```python
from build123d import *

# Parameters (mm, degrees)
BOSS_EXTRUDE1_DEPTH = 1.5


with BuildPart() as part:
    # Sketch1 → Boss-Extrude1 (new body)
    with BuildSketch(Plane(origin=(0, 0, 0), x_dir=(1, 0, 0), z_dir=(0, 1, 0))):
        with BuildLine():
            Line((15, 0), (4.75, 0))
            Line((4.75, 0), (4.75, 2))
            Line((4.75, 2), (-4.75, 2))
            Line((-4.75, 2), (-4.75, 0))
            Line((-4.75, 0), (-15, 0))
            Line((-15, 0), (-25.356589319, -6.472868325))
            ThreePointArc((-25.356589319, -6.472868325), (-27.468846161, -12.236329652), (-33.575081251, -11.609425782))
            Line((-33.575081251, -11.609425782), (-71, -35))
            Line((-71, -35), (-89.017448096, -62.257165069))
            ThreePointArc((-89.017448096, -62.257165069), (-90.820615058, -63.903738488), (-93.18854397, -64.5))
            Line((-93.18854397, -64.5), (-115.5, -64.5))
            Line((-115.5, -64.5), (-116, -65))
            Line((-116, -65), (-116, -155))
            Line((-116, -155), (-89.131068486, -155))
            ThreePointArc((-89.131068486, -155), (-86.477376272, -154.23767833), (-84.632870889, -152.183167051))
            Line((-84.632870889, -152.183167051), (-59, -99.369197466))
            Line((-59, -99.369197466), (-59, -77.369197466))
            ThreePointArc((-59, -77.369197466), (-54, -72.369197466), (-49, -77.369197466))
            Line((-49, -77.369197466), (-49, -104.800858216))
            ThreePointArc((-49, -104.800858216), (-44, -109.800858216), (-39, -104.800858216))
            Line((-39, -104.800858216), (-39, -82.800858216))
            ThreePointArc((-39, -82.800858216), (0, -43.800858216), (39, -82.800858216))
            Line((39, -82.800858216), (39, -104.800858216))
            ThreePointArc((39, -104.800858216), (44, -109.800858216), (49, -104.800858216))
            Line((49, -104.800858216), (49, -77.369197466))
            ThreePointArc((49, -77.369197466), (54, -72.369197466), (59, -77.369197466))
            Line((59, -77.369197466), (59, -99.369197466))
            Line((59, -99.369197466), (84.632870889, -152.183167051))
            ThreePointArc((84.632870889, -152.183167051), (86.477376272, -154.23767833), (89.131068486, -155))
            Line((89.131068486, -155), (116, -155))
            Line((116, -155), (116, -65))
            Line((116, -65), (115.5, -64.5))
            Line((115.5, -64.5), (93.18854397, -64.5))
            ThreePointArc((93.18854397, -64.5), (90.820615058, -63.903738488), (89.017448096, -62.257165069))
            Line((89.017448096, -62.257165069), (71, -35))
            Line((71, -35), (33.575081251, -11.609425782))
            ThreePointArc((33.575081251, -11.609425782), (27.468846161, -12.236329652), (25.356589319, -6.472868325))
            Line((25.356589319, -6.472868325), (15, 0))
        make_face()
    extrude(amount=BOSS_EXTRUDE1_DEPTH)


solid = part.part
```
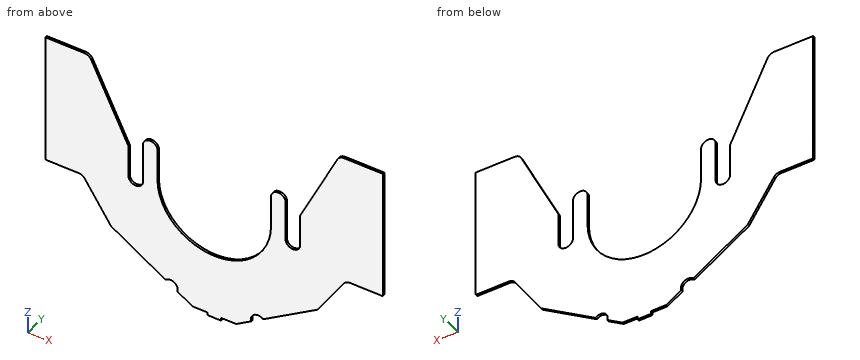
The listing builds one solid part. Answer for the finished solid, in the listing's coordinates (mm). Give positions to 0.01 mm unless a question says otherwise; leave off trailing zeros. Order: outer loops, then holes, each group sorted by start corner. A loop starts at its lowest first (then second) coordinate and runs counter-clockwise, first axis right, second up.
Item 1: The part is cut by section B-B, the plane x = 0. Give the vertices of the cut face in (y, z), and give its area (3 significant figures).
From the geometry:
outline: (0, -2) - (1.5, -2) - (1.5, 43.8) - (0, 43.8) - close
area: 68.7 mm2
Item 2: The part is cut by section C-C, the plane z = 17. Give the vertices of the cut face in (x, y), and give its area (3 significant figures).
From the geometry:
outline: (-42.2, 0) - (42.2, 0) - (42.2, 1.5) - (-42.2, 1.5) - close
area: 127 mm2
Item 3: Given pin 1 Ø0.8 at (x, y) = (9, 0.5) entering from -Z; pin 2 Ø0.8 at (y, z) = (1, -1.5) entering from -X; pin 3 Ø0.8 at (x, y) = (-107.5, 0.5) entering from -Z, each flat-ended and moving along its own axis, determine where each tip first touches the part or whether it passes through.
From the geometry:
pin 1: stops at z = 0
pin 2: stops at x = -4.75
pin 3: stops at z = 64.5
Item 4: The part is cut by section A-A, the plane z = 145.5. Give the vertices of the cut face in (x, y).
From the geometry:
outline: (-116, 0) - (-81.39, 0) - (-81.39, 1.5) - (-116, 1.5) - close; (81.39, 0) - (116, 0) - (116, 1.5) - (81.39, 1.5) - close
Item 5: Find the intervals of material crossed by probe 1 along X at (y, z) = (0.1, 102); probe 2 along X at (y, z) = (1.45, 95.5); probe 3 along X at (y, z) = (1.2, 124), in increasing order.
From the geometry:
probe 1: x = -116 to -60.28, -49 to -39, 39 to 49, 60.28 to 116
probe 2: x = -116 to -59, -49 to -39, 39 to 49, 59 to 116
probe 3: x = -116 to -70.95, 70.95 to 116
